The model under review builds one solid part; all positions refer to its coordinate system, in mm. Face numbers are marked on the shaded views. A direction names the side the tool comes from. Give positions to 0.01 mm unless a question says otherwise; leave off trailing zeros. Write each loop counter-clockwise with the first axis right and the second up, starting at its lowest first coordinate (ties: lowest second). Pieces come first, ordered by that corner, then holes. Notation, with made-up numbers: (-11, 20) - (41, 20) arc R14 ccw to (41, 40) - close; hole circle Ø5 at (3, -22). An arc over 180 degrees is marked (long way). Write item = value, one per line.
```python
from build123d import *

# Parameters (mm, degrees)
SKETCH1_W           = 39.6
SKETCH1_H           = 16.15
SKETCH1_R           = 1.8
SKETCH1_R_2         = 1.65
BOSS_EXTRUDE1_DEPTH = 1.63
SKETCH2_W           = 6.95
SKETCH2_H           = 12.5
BOSS_EXTRUDE2_DEPTH = 6
SKETCH3_W           = 11
SKETCH3_H           = 4.5
CUT_EXTRUDE1_DEPTH  = 4.65
SKETCH4_W           = 1.85
SKETCH4_H           = 0.75
SKETCH4_W_2         = 0.75
SKETCH4_H_2         = 1
CUT_EXTRUDE2_DEPTH  = 3.7
SKETCH5_W           = 0.5
SKETCH5_H           = 1.9
CUT_EXTRUDE3_DEPTH  = 6
SKETCH6_W           = 0.6
SKETCH6_H           = 0.5
BOSS_EXTRUDE3_DEPTH = 3.9
CHAMFER1_SIZE       = 0.1
BOSS_EXTRUDE4_DEPTH = 5.8
BOSS_EXTRUDE5_DEPTH = 5.8
SKETCH9_W           = 1
SKETCH9_H           = 2.8
BOSS_EXTRUDE6_DEPTH = 0.75
FILLET1_R           = 0.25
BOSS_EXTRUDE7_DEPTH = 3.65
CUT_EXTRUDE4_DEPTH  = 0.3


with BuildPart() as part:
    # Sketch1 → Boss-Extrude1 (new body)
    with BuildSketch(Plane(origin=(0, 0, 0), x_dir=(1, 0, 0), z_dir=(0, 1, 0))):
        Rectangle(SKETCH1_W, SKETCH1_H)
        with Locations(Location((-17.3, 5.575, 0), (0, 0, 270))):
            Circle(SKETCH1_R, mode=Mode.SUBTRACT)
        with Locations(Location((-17.3, -5.575, 0), (0, 0, 270))):
            Circle(SKETCH1_R, mode=Mode.SUBTRACT)
        with Locations(Location((-2.45, 5.325, 0), (0, 0, 270))):
            Circle(SKETCH1_R_2, mode=Mode.SUBTRACT)
        with Locations(Location((16.55, 5.325, 0), (0, 0, 270))):
            Circle(SKETCH1_R_2, mode=Mode.SUBTRACT)
    extrude(amount=BOSS_EXTRUDE1_DEPTH)

    # Sketch2 → Boss-Extrude2 (add)
    with BuildSketch(Plane(origin=(0, 1.63, 0), x_dir=(1, 0, 0), z_dir=(0, 1, 0))):
        with Locations((-12.175, 0)):
            Rectangle(SKETCH2_W, SKETCH2_H)
    extrude(amount=BOSS_EXTRUDE2_DEPTH)

    # Sketch3 → Cut-Extrude1 (cut)
    with BuildSketch(Plane.ZY.offset(15.65)):
        with Locations((0, 4.63)):
            Rectangle(SKETCH3_W, SKETCH3_H)
    extrude(amount=-CUT_EXTRUDE1_DEPTH, mode=Mode.SUBTRACT)

    # Sketch4 → Cut-Extrude2 (cut)
    with BuildSketch(Plane.ZY.offset(15.65)):
        with Locations((-3.525, 7.255)):
            Rectangle(SKETCH4_W, SKETCH4_H)
        with Locations((-5.875, 6.38)):
            Rectangle(SKETCH4_W_2, SKETCH4_H_2)
        with Locations((5.875, 6.38)):
            Rectangle(SKETCH4_W_2, SKETCH4_H_2)
        with Locations((3.525, 7.255)):
            Rectangle(SKETCH4_W, SKETCH4_H)
    extrude(amount=-CUT_EXTRUDE2_DEPTH, mode=Mode.SUBTRACT)

    # Sketch5 → Cut-Extrude3 (cut)
    with BuildSketch(Plane(origin=(0, 7.63, 0), x_dir=(1, 0, 0), z_dir=(0, 1, 0))):
        with Locations((-8.95, 3.8)):
            Rectangle(SKETCH5_W, SKETCH5_H)
        with Locations((-8.95, 1.26)):
            Rectangle(SKETCH5_W, SKETCH5_H)
        with Locations((-8.95, -1.28)):
            Rectangle(SKETCH5_W, SKETCH5_H)
        with Locations((-8.95, -3.82)):
            Rectangle(SKETCH5_W, SKETCH5_H)
    extrude(amount=-CUT_EXTRUDE3_DEPTH, mode=Mode.SUBTRACT)

    # Sketch6 → Boss-Extrude3 (add)
    with BuildSketch(Plane.ZY.offset(11)):
        with Locations((-3.8, 5.38)):
            Rectangle(SKETCH6_W, SKETCH6_H)
        with Locations((-1.26, 5.38)):
            Rectangle(SKETCH6_W, SKETCH6_H)
        with Locations((1.28, 5.38)):
            Rectangle(SKETCH6_W, SKETCH6_H)
        with Locations((3.82, 5.38)):
            Rectangle(SKETCH6_W, SKETCH6_H)
    extrude(amount=BOSS_EXTRUDE3_DEPTH)

    # Chamfer1
    chamfer1_edges = [part.edges().sort_by_distance(p)[0] for p in [
        (-14.9, 5.38, -4.1),
        (-14.9, 5.13, -3.8),
        (-14.9, 5.38, -3.5),
        (-14.9, 5.63, -3.8),
        (-14.9, 5.63, -1.26),
        (-14.9, 5.38, -1.56),
        (-14.9, 5.13, -1.26),
        (-14.9, 5.38, -0.96),
        (-14.9, 5.63, 1.28),
        (-14.9, 5.38, 0.98),
        (-14.9, 5.13, 1.28),
        (-14.9, 5.38, 1.58),
        (-14.9, 5.63, 3.82),
        (-14.9, 5.38, 3.52),
        (-14.9, 5.13, 3.82),
        (-14.9, 5.38, 4.12),
    ]]
    chamfer(chamfer1_edges, length=CHAMFER1_SIZE)

    # Sketch7 → Boss-Extrude4 (add)
    with BuildSketch(Plane(origin=(0, 1.63, 0), x_dir=(1, 0, 0), z_dir=(0, 1, 0))):
        Polygon((0.5, 7.575), (13.3, 7.575), (13.3, 4.325), (8.7, 4.325), (8.7, 2.375), (5.1, 2.375), (5.1, 4.325), (0.5, 4.325), align=None)
    extrude(amount=BOSS_EXTRUDE4_DEPTH)

    # Sketch8 → Boss-Extrude5 (add)
    with BuildSketch(Plane(origin=(0, 1.63, 0), x_dir=(1, 0, 0), z_dir=(0, 1, 0))):
        Polygon((0.5, 4.324), (0.5, 2.025), (13.3, 2.025), (13.3, 4.324), (8.701, 4.324), (8.701, 2.374), (5.099, 2.374), (5.099, 4.324), align=None)
    extrude(amount=BOSS_EXTRUDE5_DEPTH)

    # Sketch9 → Boss-Extrude6 (add)
    with BuildSketch(Plane(origin=(0, 0, -7.575), x_dir=(-1, 0, 0), z_dir=(0, 0, -1))):
        with Locations((-4.8, 4.53)):
            Rectangle(SKETCH9_W, SKETCH9_H)
    extrude(amount=BOSS_EXTRUDE6_DEPTH)

    # Fillet1
    fillet1_edges = [part.edges().sort_by_distance(p)[0] for p in [
        (4.3, 4.53, -8.325),
        (5.3, 4.53, -8.325),
    ]]
    fillet(fillet1_edges, radius=FILLET1_R)

    # Sketch10 → Boss-Extrude7 (add)
    with BuildSketch(Plane(origin=(0, 2.88, 0), x_dir=(1, 0, 0), z_dir=(0, 1, 0))):
        with BuildLine():
            ThreePointArc((1.986591762, 7.65728792), (1.960185355, 7.63936483), (1.95, 7.609119267))
            Line((1.95, 7.609119267), (1.95, 7.575))
            Line((1.95, 7.575), (1.65, 7.575))
            Line((1.65, 7.575), (1.65, 7.685085191))
            ThreePointArc((1.65, 7.685085191), (1.700926776, 7.836313004), (1.832958812, 7.925928458))
            Line((1.832958812, 7.925928458), (13.03488517, 11.044099284))
            ThreePointArc((13.03488517, 11.044099284), (13.164742187, 11.130893542), (13.217742469, 11.277818891))
            ThreePointArc((13.217742469, 11.277818891), (14.51265049, 12.6340191), (15.995064384, 11.485753085))
            ThreePointArc((15.995064384, 11.485753085), (15.976497018, 11.407856176), (15.906722272, 11.368560369))
            Line((15.906722272, 11.368560369), (15.806911036, 11.35844928))
            ThreePointArc((15.806911036, 11.35844928), (15.736894481, 11.377893571), (15.698527539, 11.439605615))
            ThreePointArc((15.698527539, 11.439605615), (14.474302897, 12.328608683), (13.520358774, 11.154282051))
            Line((13.520358774, 11.154282051), (13.502671925, 11.020626045))
            ThreePointArc((13.502671925, 11.020626045), (13.443534072, 10.889435933), (13.321873718, 10.812579642))
            Line((13.321873718, 10.812579642), (1.986591762, 7.65728792))
        make_face()
    extrude(amount=BOSS_EXTRUDE7_DEPTH)

    # Sketch11 → Cut-Extrude4 (cut)
    with BuildSketch(Plane(origin=(1.123559568, 0, -7.728459919), x_dir=(0.9633730670576666, 0, -0.26816475097951425), z_dir=(0.26816475097951425, 0, 0.9633730670576666))):
        with BuildLine():
            Line((0.466005992, 5.13), (8.136005992, 5.13))
            ThreePointArc((8.136005992, 5.13), (8.561005992, 4.705), (8.136005992, 4.28))
            Line((8.136005992, 4.28), (0.466005992, 4.28))
            Line((0.466005992, 4.28), (0.466005992, 5.13))
        make_face()
    extrude(amount=CUT_EXTRUDE4_DEPTH, mode=Mode.SUBTRACT)


solid = part.part
```
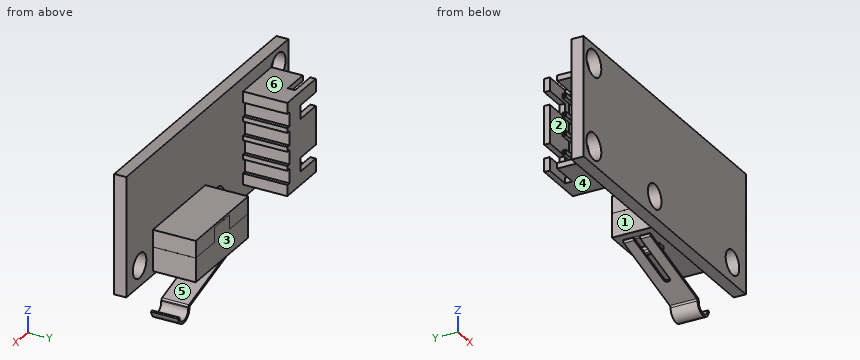
1. Insertion check: P1, Ø0.6, axis at x = -13.5, y = 5.5, coming from the +Z side; P2, Ø5, axis at x = -3.5, z = 5.5, coming from the +Y side; P3, Ø0.8, axis at y = 7, z = 5, coming from the -X side. Each pin has a flat end and moves straight along its axis. Give the tip position at first contact, or say it passes through.
Findings below:
P1 = 6.25
P2 = 1.63
P3 = -15.65
2. Take a section at B-B on y = 1.25. Give the boundary of the cut face in (x, z) (3 decimals), and give its area (3 significant figures).
Findings below:
outline = (-19.8, -8.075) - (19.8, -8.075) - (19.8, 8.075) - (-19.8, 8.075) - close; hole circle Ø3.6 at (-17.3, -5.575); hole circle Ø3.6 at (-17.3, 5.575); hole circle Ø3.3 at (-2.45, -5.325); hole circle Ø3.3 at (16.55, -5.325)
area = 602 mm²
3. Take a section at D-D on x = 2.5. Count the separate pieces of the cut face and the enclosed holes in it, and give its area (3 significant figures).
Findings below:
separate_pieces = 3
enclosed_holes = 0
area = 59.4 mm²
4. Machinability: for the marked faces 1, 2 and 3, which of the approach directions +Z, -Z, +X, -X, +Y, -Y give a long, thin tool a straight path to every point of the face, cutting with its end or side? Answer none if there is none.
Findings below:
face_1 = +Z, -Z, +Y
face_2 = -X
face_3 = +Z, -Z, +X, +Y
5. For line 1 (Z direction, x = -17.3, y = 0.5) (3 decimals); line 2 (X direction, y = 1.25, z = -6); line 3 (Z direction, x = -12, y = 5), list the stretches that pass through material, from the lowest coordinate up. Write a range as from..to.
Findings below:
line_1 = -8.075..-7.375, -3.775..3.775, 7.375..8.075
line_2 = -19.8..-19.05, -15.55..-3.96, -0.94..15.04, 18.06..19.8
line_3 = -6.25..-5.5, 5.5..6.25
6. Take a section at C-C on x = 16.55. Give the boundary of the cut face in (y, z) (3 decimals), and give its area (3 significant figures).
Findings below:
outline = (0, -8.075) - (1.63, -8.075) - (1.63, -6.975) - (0, -6.975) - close; (0, -3.675) - (1.63, -3.675) - (1.63, 8.075) - (0, 8.075) - close
area = 20.9 mm²
7. Draft analysis for pull direction Z (two halves, no side actions). For the marked faces 4, 5 and 6, state which applies: +Z half, -Z half, draft (parallel to the pull), parting line (faces both ways), or undercut.
Findings below:
face_4 = -Z half
face_5 = undercut
face_6 = +Z half
8. Take a section at A-A on x = -17.3. Give the boundary of the cut face in (y, z) (3 decimals).
Findings below:
outline = (0, -8.075) - (1.63, -8.075) - (1.63, -7.375) - (0, -7.375) - close; (0, -3.775) - (1.63, -3.775) - (1.63, 3.775) - (0, 3.775) - close; (0, 7.375) - (1.63, 7.375) - (1.63, 8.075) - (0, 8.075) - close
